```python
from build123d import *

# Parameters (mm, degrees)
ESQUISSE1_W             = 6
ESQUISSE1_H             = 6
ESQUISSE1_W_2           = 4
ESQUISSE1_H_2           = 4
BOSS_EXTRU_1_DEPTH      = 10
ESQUISSE2_W             = 2
ESQUISSE2_H             = 2
BOSS_EXTRU_2_DEPTH      = 4
BOSS_EXTRU_2_DEPTH_BACK = 6
ESQUISSE4_R             = 2.5
ESQUISSE4_R_2           = 2


with BuildPart() as part:
    # Esquisse1 → Boss.-Extru.1 (new body)
    with BuildSketch(Plane.XY):
        Rectangle(ESQUISSE1_W, ESQUISSE1_H)
        Rectangle(ESQUISSE1_W_2, ESQUISSE1_H_2, mode=Mode.SUBTRACT)
    extrude(amount=BOSS_EXTRU_1_DEPTH)

    # Balayage1: sweep along a path in Esquisse3
    with BuildLine(Plane(origin=(0, 0, 0), x_dir=(0, 0, -1), z_dir=(1, 0, 0))) as balayage1_path:
        Line((-5, 3), (-5, 18))
        ThreePointArc((-5, 18), (-5.585786438, 19.414213562), (-7, 20))
        Line((-7, 20), (-32, 20))
    # Esquisse2 → Balayage1 (sweep)
    with BuildSketch(Plane(origin=(0, 3, 0), x_dir=(1, 0, 0), z_dir=(0, 1, 0))):
        with Locations((0, -5)):
            Rectangle(ESQUISSE2_W, ESQUISSE2_H)
    sweep(path=balayage1_path.line)

    # Esquisse4 → Boss.-Extru.2 (add, two sides: drawn at the far end of the back side and taken through both)
    with BuildSketch(Plane.XZ.offset(-19).offset(-BOSS_EXTRU_2_DEPTH_BACK)):
        with Locations(Location((0, 34, 0), (0, 0, 270))):
            Circle(ESQUISSE4_R)
        with Locations(Location((0, 34, 0), (0, 0, 270))):
            Circle(ESQUISSE4_R_2, mode=Mode.SUBTRACT)
    extrude(amount=BOSS_EXTRU_2_DEPTH + BOSS_EXTRU_2_DEPTH_BACK)


solid = part.part
```
Verification items for the finished model (mm, model axes). A direction names the side the tool comes from. Coordinates: 2 decimals unless noted, no trailing zeros. Loops run counter-clockwise (first coordinate to the right, second up) from the corner with the lowest first, then second, coordinate; pieces in that order, holes last. Notation, with made-up numbers: (26, 9.25) -> (75, 9.25) arc R20 ccw to (75, 35.25) -> close; hole circle Ø3 at (85, 7). An arc over 180 degrees is marked (long way). Answer in a Markdown table with one row per item.
1) Depth check by flat-ended pin: P1, Ø1.6, axis at x = 0, y = 8.5, coming from the -Z side; P2, Ø3, axis at x = 1.5, z = 21, coming from the -Y side; P3, Ø1.5, axis at x = -1, z = 11, coming from the +Y side; P4, Ø2.5, axis at x = 0, z = 34, coming from the -Y side. Enter the tip coordinate at first touch or a pass-through.
The answers:
| item | result |
|---|---|
| P1 | stops at z = 4 |
| P2 | stops at y = 19 |
| P3 | stops at y = 21 |
| P4 | passes through |
2) Access from +Z, -Z, +X, -X, +Y, -Y to the whole of each face (thin tool, end or side, straight path). Record for faces 4 (the face through (0, 11, 6)), 5 (the face through (0, 2, 5)), 6 (the face through (2, 15, 35)), 7 (the face through (0, 11, 4)), 8 (the face through (-1, 19.4, 11.6)).
The answers:
| item | result |
|---|---|
| face 4 | +X, -X |
| face 5 | +Z, -Z |
| face 6 | +Z, +X, -X, -Y |
| face 7 | -Z, +X, -X, +Y |
| face 8 | -Z, -X, +Y |
3) Draft check along X on faces 1 (the face through (0.1, 20.1, 36.5)), 2 (the face through (0, 19, 20)), 3 (the face through (0, -2, 5)). Enter one of: released by +X, released by -X, zero draft, split by the parting line, or undercut.
The answers:
| item | result |
|---|---|
| face 1 | split by the parting line |
| face 2 | zero draft |
| face 3 | undercut |
4) Section check C-C (z = 20). Record the cut outline in (x, y), and give its area (3 significant figures).
The answers:
| item | result |
|---|---|
| outline | (-1, 19) -> (1, 19) -> (1, 21) -> (-1, 21) -> close |
| area | 4.00 mm2 |
5) Section check B-B (z = 34). Record the cut outline in (x, y), and give its area (3 significant figures).
The answers:
| item | result |
|---|---|
| outline | (-2.5, 15) -> (-2, 15) -> (-2, 25) -> (-2.5, 25) -> close; (2, 15) -> (2.5, 15) -> (2.5, 25) -> (2, 25) -> close |
| area | 10.0 mm2 |
6) Section check A-A (x = 0). Record the cut outline in (y, z), and give its area (3 significant figures).
The answers:
| item | result |
|---|---|
| outline | (-3, 0) -> (-2, 0) -> (-2, 10) -> (-3, 10) -> close; (2, 0) -> (3, 0) -> (3, 4) -> (18, 4) arc R3 ccw to (21, 7) -> (21, 31.5) -> (25, 31.5) -> (25, 32) -> (15, 32) -> (15, 31.5) -> (19, 31.5) -> (19, 7) arc R1 cw to (18, 6) -> (3, 6) -> (3, 10) -> (2, 10) -> close; (15, 36) -> (25, 36) -> (25, 36.5) -> (15, 36.5) -> close |
| area | 115 mm2 |
7) Scan lines: line 1 along X through (y, z) = (20.75, 34); line 2 along Y through (x, z) = (-0.8, 11.5); line 3 along Z through (x, y) = (2.6, 0.25). Record each from-to range of solid material in increasing order. Write a range as from..to.
The answers:
| item | result |
|---|---|
| line 1 | x = -2.5..-2, 2..2.5 |
| line 2 | y = 19..21 |
| line 3 | z = 0..10 |
